Source: CAD feature listing. Evaluate the final solid. Frame: model axes, mm. Face numbers are marked on the shaded views. A direction names the side the tool comes from. Coordinates: 2 decimals unless noted, no trailing zeros. Write each loop counter-clockwise with the first axis right and the second up, starting at its lowest first coordinate (ties: lowest second). Pieces come first, ordered by that corner, then holes. Notation, with made-up numbers: (47.5, 72.25) -> (104.5, 72.25) arc R13 cw to (104.5, 80.25) -> close; hole circle Ø2 at (25, 54.25). An arc over 180 degrees is marked (long way). Write item = value, one per line.
from build123d import *

# Parameters (mm, degrees)
F0_W     = 50
F0_H     = 2.5
F0_H_2   = 22
F1_DEPTH = 2.5
F2_DEPTH = 5
F3_W     = 50
F3_H     = 2.5
F4_DEPTH = 2
F5_DEPTH = 5.5
F6_W     = 50
F6_H     = 2.5
F7_DEPTH = 1.5
F8_SIZE  = 2


with BuildPart() as f1:
    # F0 (on Top) → F1 (new body)
    with BuildSketch(Plane.XY):
        with Locations((0, 14.75)):
            Rectangle(F0_W, F0_H)
        with Locations((0, 12.25)):
            Rectangle(F0_W, F0_H)
        Rectangle(F0_W, F0_H_2)
        with Locations((0, -12.25)):
            Rectangle(F0_W, F0_H)
        with Locations((0, -14.75)):
            Rectangle(F0_W, F0_H)
    extrude(amount=F1_DEPTH)

    # F0 (on Top) → F2 (join)
    with BuildSketch(Plane.XY):
        with Locations((0, -12.25)):
            Rectangle(F0_W, F0_H)
    extrude(amount=-F2_DEPTH)

    # F3 (on face) → F4 (join)
    with BuildSketch(Plane.XZ.offset(13.5)):
        with Locations((0, -3.75)):
            Rectangle(F3_W, F3_H)
    extrude(amount=F4_DEPTH)

    # F0 (on Top) → F5 (join)
    with BuildSketch(Plane.XY):
        with Locations((0, 12.25)):
            Rectangle(F0_W, F0_H)
    extrude(amount=-F5_DEPTH)

    # F6 (on face) → F7 (join)
    with BuildSketch(Plane(origin=(0, 13.5, 0), x_dir=(-1, 0, 0), z_dir=(0, 1, 0))):
        with Locations((0, -4.25)):
            Rectangle(F6_W, F6_H)
    extrude(amount=F7_DEPTH)

    # F8
    f8_edges = [f1.edges().sort_by_distance(p)[0] for p in [
        (0, 15, -5.5),
    ]]
    chamfer(f8_edges, length=F8_SIZE)


solid = f1.part
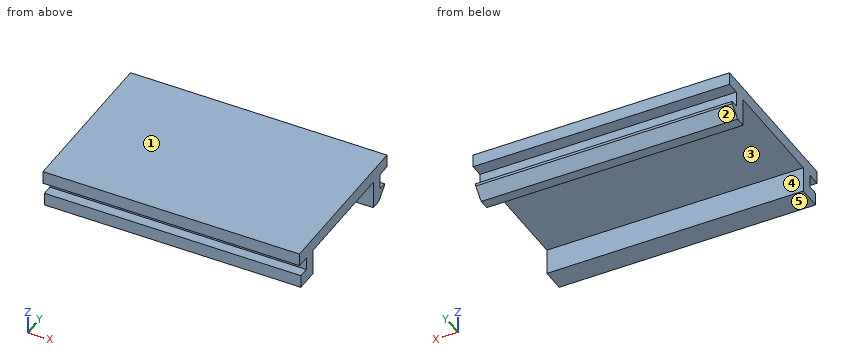
1) Reachability of the marked faces 4 and 5 from +Z, -Z, +X, -X, +Y, -Y: full face, straight path, thin tool, end or side. Return the list, or none.
Answer block:
face_4 = -Z, +X, -X
face_5 = -Z, +X, -X, -Y
2) Cut plane A-A, the plane z = -4.5. Output: boundary loops of the cut face in (x, y).
Answer block:
outline = (-25, -15.5) -> (25, -15.5) -> (25, -11) -> (-25, -11) -> close; (-25, 11) -> (25, 11) -> (25, 14) -> (-25, 14) -> close
3) Pull-direction query (Y, two-part tool) for the marked faces 1, 2 and 3; classes: +Y half, -Y half, draft (parallel to the pull), parting line (faces both ways), or undercut.
Answer block:
face_1 = draft
face_2 = +Y half
face_3 = undercut
4) Cut plane D-D, the plane y = -12. Output: boundary loops of the cut face in (x, z), and give its area (3 significant figures).
Answer block:
outline = (-25, -5) -> (25, -5) -> (25, 2.5) -> (-25, 2.5) -> close
area = 375 mm2
5) Cut plane C-C, the plane z = -1.5. Output: boundary loops of the cut face in (x, y), and give its area (3 significant figures).
Answer block:
outline = (-25, -13.5) -> (25, -13.5) -> (25, -11) -> (-25, -11) -> close; (-25, 11) -> (25, 11) -> (25, 13.5) -> (-25, 13.5) -> close
area = 250 mm2
6) Material intervals for probe 1 along Y at (x, z) = (6, -2.75); probe 2 along Y at (x, z) = (1, -0.75); probe 3 along Z at (x, y) = (-18, 8), sorted ascending. Write a range as [from, to].
Answer block:
probe_1 = [-15.5, -11], [11, 13.5]
probe_2 = [-13.5, -11], [11, 13.5]
probe_3 = [0, 2.5]
7) Cut plane B-B, the plane x = 10. Output: boundary loops of the cut face in (y, z), and give its area (3 significant figures).
Answer block:
outline = (-16, 0) -> (-13.5, 0) -> (-13.5, -2.5) -> (-15.5, -2.5) -> (-15.5, -5) -> (-11, -5) -> (-11, 0) -> (11, 0) -> (11, -5.5) -> (13, -5.5) -> (15, -3.5) -> (15, -3) -> (13.5, -3) -> (13.5, 0) -> (16, 0) -> (16, 2.5) -> (-16, 2.5) -> close
area = 113 mm2
8) First-contact query: pin 1 Ø1.5 at (x, z) = (3, -2) entering from +Y; pin 2 Ø2 at (x, y) = (-11.5, 15) entering from -Z; pin 3 Ø1.2 at (x, y) = (-6, -15.5) entering from -Z. Flat tips, straight axial feed; report the tip coordinate or a pass-through.
Answer block:
pin_1 = 13.5
pin_2 = -4.5
pin_3 = -5
